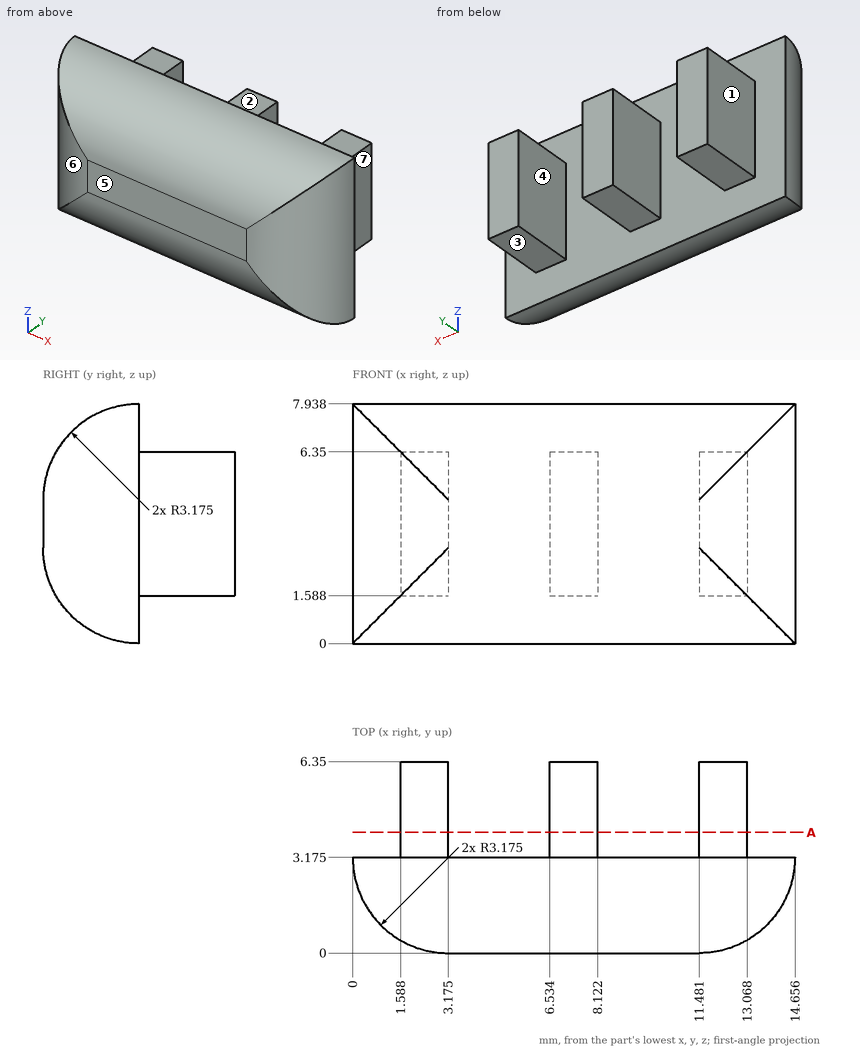
Can you work these out from the drawing? Everything is in mm from the part's minimum corner. A direction names the side the tool comes from. Give positions to 0.01 mm unless a question says otherwise; leave off trailing zeros. Use CSV: the item, a comma, the result in double quotes. Start each with the question number.
1. For P1, Ø0.5, axis at x = 7.5, y = 4.5, coming from the -Z side; P2, Ø2.5, axis at y = 4.5, z = 5, coming from the +X side; P3, Ø0.8, axis at x = 7, y = 4.5, coming from the +Z side, each with a flat end and sliding along its axis, tell me the tip position at first contact or that it passes through.
2. Imagine slicing it at A-A, the plane y = 4. Count the separate pieces of the cut face and the enclosed holes in it.
3. If we mould it in two halves opening along X, with no side actions, what happens to the marked faces 4, 5, 6 and 7? For each: released by +X, released by -X, zero draft, split by the parting line, or undercut.
4. On a 3-axis mill with a long thin cutter (end or side, diameter ignored), from which of +Z, -Z, +X, -X, +Y, -Y can I reach the whole of each face in a straight line? I mean the marked faces 1, 2 and 3. Say none if no direction works.
5. If I drill on L1, parallel to X at y = 5.5, z = 4 (1 decimal); L2, parallel to Y at x = 9, z = 4 (1 decimal); L3, parallel to Z at x = 3, y = 5, over which ranges is the centre line in solid material (lowest first)?
Response values:
1,P1,"z = 1.59"
1,P2,"x = 13.07"
1,P3,"z = 6.35"
2,separate pieces,"3"
2,enclosed holes,"0"
3,face 4,"undercut"
3,face 5,"zero draft"
3,face 6,"released by -X"
3,face 7,"released by +X"
4,face 1,"+Z, -Z, -X, +Y"
4,face 2,"+Z, +X, -X, +Y"
4,face 3,"-Z, +X, -X, +Y"
5,L1,"1.6 to 3.2, 6.5 to 8.1, 11.5 to 13.1"
5,L2,"0 to 3.2"
5,L3,"1.59 to 6.35"
